from build123d import *

# Parameters (mm, degrees)
SKETCH1_R               = 4.7625
BOSS_EXTRUDE1_DEPTH     = 5.08
SKETCH4_W               = 19.05
SKETCH4_H               = 5.08
BOSS_EXTRUDE2_DEPTH     = 5.08
SKETCH6_R               = 4.7625
BOSS_EXTRUDE3_DEPTH     = 5.08
SKETCH8_R               = 4.7625
CUT_EXTRUDE2_DEPTH      = 6.0800001
SKETCH5_R               = 1.651
SKETCH5_R_2             = 1.660728382
CUT_EXTRUDE1_DEPTH      = 1.0000001
CUT_EXTRUDE1_DEPTH_BACK = 6.0800001


with BuildPart() as part:
    # Sketch1 → Boss-Extrude1 (new body)
    with BuildSketch(Plane(origin=(0, 0, 0), x_dir=(1, 0, 0), z_dir=(0, 1, 0))):
        with BuildLine():
            Line((-9.525, 53.975), (9.525, 53.975))
            Line((9.525, 53.975), (9.525, 51.435))
            add(Edge.make_bspline(
                [(9.525, 51.435), (9.525, 51.21454564), (27.819109584, -48.895), (60.325, -48.895)],
                knots=[0, 0, 0, 0, 1, 1, 1, 1], degree=3))
            Line((60.325, -48.895), (-9.525, -48.895))
            Line((-9.525, -48.895), (-9.525, 53.975))
        make_face()
        with Locations((0, 45.9867)):
            Circle(SKETCH1_R, mode=Mode.SUBTRACT)
    extrude(amount=BOSS_EXTRUDE1_DEPTH)

    # Sketch4 → Boss-Extrude2 (add)
    with BuildSketch(Plane(origin=(0, 5.08, 0), x_dir=(1, 0, 0), z_dir=(0, 1, 0))):
        with Locations((50.8, -51.435)):
            Rectangle(SKETCH4_W, SKETCH4_H)
    extrude(amount=-BOSS_EXTRUDE2_DEPTH)

    # Sketch6 → Boss-Extrude3 (add)
    with BuildSketch(Plane.XZ):
        with BuildLine():
            Line((-13.5128, 12.403582), (-9.525, 12.403582))
            Line((-9.525, 12.403582), (-9.525, 11.565453148))
            ThreePointArc((-9.525, 11.565453148), (-3.6068, 2.497582), (-9.525, -6.570289148))
            Line((-9.525, -6.570289148), (-9.525, -7.408418))
            Line((-9.525, -7.408418), (-13.5128, -7.408418))
            ThreePointArc((-13.5128, -7.408418), (-23.4188, 2.497582), (-13.5128, 12.403582))
        make_face()
        with Locations((-13.5128, 2.497582)):
            Circle(SKETCH6_R, mode=Mode.SUBTRACT)
    extrude(amount=-BOSS_EXTRUDE3_DEPTH)

    # Sketch8 → Cut-Extrude2 (cut, through all)
    with BuildSketch(Plane(origin=(0, 5.08, 0), x_dir=(1, 0, 0), z_dir=(0, 1, 0))):
        with Locations((-13.5128, -2.497582)):
            Circle(SKETCH8_R)
    extrude(amount=-CUT_EXTRUDE2_DEPTH, mode=Mode.SUBTRACT)

    # Sketch5 → Cut-Extrude1 (cut, two sides)
    with BuildSketch(Plane.XZ) as cut_extrude1_sk:
        with Locations((34.925, 40.005)):
            Circle(SKETCH5_R)
        with Locations((-3.175, 4.445)):
            Circle(SKETCH5_R_2)
    extrude(amount=CUT_EXTRUDE1_DEPTH, mode=Mode.SUBTRACT)
    extrude(cut_extrude1_sk.sketch, amount=-CUT_EXTRUDE1_DEPTH_BACK, mode=Mode.SUBTRACT)


solid = part.part
Model file for the job. Use its own axes, mm. A direction names the side the tool comes from. Round coordinates to 2 decimals unless told otherwise and drop trailing zeros. Loops run counter-clockwise (first coordinate to the right, second up) from the corner with the lowest first, then second, coordinate; pieces in that order, holes last. Notation, with made-up numbers: (-11.75, -15.75) - (11.25, -15.75) arc R33 cw to (11.25, 14.25) - close; hole circle Ø3 at (-15, 78.25). An arc over 180 degrees is marked (long way). Write each question's results on one line, items separated by ' | '.
(1) 3-axis set-ups, long thin cutter, end or side, ignore diameter. For faces 4 (the flat face through (10, 5.08, 13)), 5 (the flat face through (9.525, 3, -53)), 6 (the flat face through (-12, 3, 12.404)), 7 (the flat face through (-11, 3, -7.408)): which of +Z, -Z, +X, -X, +Y, -Y reach the whole face in a straight line?
Answer below:
face 4: +Z, -Z, +X, -X, +Y | face 5: -Z, +X, +Y, -Y | face 6: +Z, -X, +Y, -Y | face 7: -Z, -X, +Y, -Y
(2) Saw through at A-A, the plane x = 0. List the corners of the cut face in (y, z) (3 decimals).
Answer below:
outline: (0, -53.975) - (5.08, -53.975) - (5.08, -50.749) - (0, -50.749) - close; (0, -41.224) - (5.08, -41.224) - (5.08, 48.895) - (0, 48.895) - close
(3) Mould opens along Z. For faces 1 (the cylindrical face through (-1.59, 2.5, 4.94)), 2 (the flat face through (-9.525, 3, -30)), 3 (the flat face through (51, 3, 53.975)) say: released by +Z, released by -Z, zero draft, split by the parting line, or undercut.
Answer below:
face 1: undercut | face 2: zero draft | face 3: released by +Z
(4) Wall check: L1, parallel to X at y = 3.55, z = 3; L2, parallel to Z at x = 36, y = 1.9 (3 decimals); L3, parallel to X at y = 2.8, z = -1.5. Give the ranges that are in metal, low to high.
Answer below:
L1: x = -23.41 to -18.25, -8.78 to -3.99, -2.36 to 24.22 | L2: z = 28.978 to 38.752, 41.258 to 48.895 | L3: x = -22.58 to -16.1, -10.92 to 22.63
(5) Pin check, flat tips, straight feed: pin 1 (1.5 mm diameter, centred on x = 20, y = 1.5, fed in from +Z) (3 decimals); pin 2 (2.5 mm diameter, centred on y = 1.5, z = -31.5, fed in from -X) (3 decimals); pin 3 (3 mm diameter, centred on x = 51, y = 1, fed in from -Z). Stop position of each tip, or through.
Answer below:
pin 1: stops at z = 48.895 | pin 2: stops at x = -9.525 | pin 3: stops at z = 45.1
(6) Saw through at B-B, the plane y = 3.2. Count the separate pieces of the cut face and the enclosed holes in it, then the cut area to 3 significant figures.
Answer below:
separate pieces: 1 | enclosed holes: 4 | area: 3,700 mm^2
